```python
from build123d import *

# Parameters (mm, degrees)
F0_W     = 55.156417
F0_H     = 77.16199
F1_DEPTH = 25.4
F3_D     = 25.4
F4_W     = 25.4
F4_H     = 25.4
F5_DEPTH = 12.7


with BuildPart() as f1:
    # F0 (on Top) → F1 (new body)
    with BuildSketch(Plane.XY):
        with Locations((-27.578208, 38.580995)):
            Rectangle(F0_W, F0_H)
    extrude(amount=F1_DEPTH)

    # F3 (through all)
    with Locations(Plane.XY.offset(25.4)):
        with Locations((-30.758334, 40.183466)):
            Hole(F3_D / 2)

    # F4 (on face) → F5 (join)
    with BuildSketch(Plane.XZ):
        with Locations((-12.898058, 23.184226)):
            Rectangle(F4_W, F4_H)
    extrude(amount=F5_DEPTH)


solid = f1.part
```
Verification items for the finished model (mm, model axes). A direction names the side the tool comes from. Coordinates: 2 decimals unless noted, no trailing zeros. Write each loop counter-clockwise with the first axis right and the second up, starting at its lowest first coordinate (ties: lowest second). Pieces come first, ordered by that corner, then holes. Notation, with made-up numbers: (54.25, -12.5) - (89.25, -12.5) arc R18 ccw to (89.25, 22.5) - close; hole circle Ø5 at (-29.5, 27.5). An arc over 180 degrees is marked (long way). Write item = value, one per line.
Q1. Cross-section at C-C (x = -11). Enter the section's corners in (y, z).
Answer:
outline = (-12.7, 10.48) - (0, 10.48) - (0, 0) - (77.16, 0) - (77.16, 25.4) - (0, 25.4) - (0, 35.88) - (-12.7, 35.88) - close
Q2. Cross-section at A-A (x = -38). Enter the section's corners in (y, z), plus the area to 3 significant figures.
Answer:
outline = (0, 0) - (29.75, 0) - (29.75, 25.4) - (0, 25.4) - close; (50.62, 0) - (77.16, 0) - (77.16, 25.4) - (50.62, 25.4) - close
area = 1,430 mm²
Q3. Access from +Z, -Z, +X, -X, +Y, -Y to the whole of each face (thin tool, end or side, straight path). Record for faces 1 (the face through (-13, -6, 10.484)), 2 (the face through (-21.8, 30.5, 25.4)), 3 (the face through (-25.598, -6, 23)), 4 (the face through (-0.198, -6, 23)), 5 (the face through (0, 38, 13)).
Answer:
face_1 = -Z, +X, -X, -Y
face_2 = +Z, +X, -X, +Y
face_3 = +Z, -Z, -X, -Y
face_4 = +Z, -Z, +X, -Y
face_5 = +Z, -Z, +X, +Y, -Y
Q4. Go/stop test with flat-tipped pins: pin 1 Ø4 at (x, y) = (-14, -4) entering from -Z; pin 2 Ø6 at (x, y) = (-24, 59.5) entering from +Z; pin 3 Ø4 at (y, z) = (-8.5, 22) entering from -X. Record where each tip stops, or that it passes through.
Answer:
pin_1 = 10.48
pin_2 = 25.4
pin_3 = -25.6
Q5. Cross-section at B-B (y = 51). Enter the section's corners in (x, z).
Answer:
outline = (-55.16, 0) - (-37.41, 0) - (-37.41, 25.4) - (-55.16, 25.4) - close; (-24.1, 0) - (0, 0) - (0, 25.4) - (-24.1, 25.4) - close
Q6. Material ranges on L1, parallel to Z at x = -5.5, y = 55; L2, parallel to Y at x = -34, z = 22; L3, parallel to Y at x = -45, z = 25, recorded low to high. Write a range as from..to.
Answer:
L1 = 0..25.4
L2 = 0..27.9, 52.46..77.16
L3 = 0..77.16
Q7. Cross-section at D-D (z = 27). Enter the section's corners in (x, y).
Answer:
outline = (-25.6, -12.7) - (-0.2, -12.7) - (-0.2, 0) - (-25.6, 0) - close
Q8. Mould release check, pull along Y, two halves, no side actions. Record for faces 6 (the face through (-37.59, 50.89, 12.52)), 7 (the face through (-13, -6, 35.884)), 8 (the face through (-13, 0, 31)): released by +Y, released by -Y, zero draft, split by the parting line, or undercut.
Answer:
face_6 = undercut
face_7 = zero draft
face_8 = released by +Y
